Read the model definition and answer for the solid it produces. Units are mm, in the model's axes. Round coordinates to 2 decimals unless told otherwise and drop trailing zeros. Order: outer loops, then holes, each group sorted by start corner. A loop starts at its lowest first (then second) coordinate and runs counter-clockwise, first axis right, second up. Notation, with made-up numbers: (3.25, 62) - (57.25, 62) arc R23 ccw to (57.25, 85) - close; hole circle Ø6 at (61.25, -18). An arc over 180 degrees is marked (long way). Answer as a JSON object with one key per item and string values. Group by question number.
Q1. A cutting plane is placed at B-B on x = -267. Determine the outline of the cut face in (y, z).
Q2. Given pin 1 Ø22.5 at (y, z) = (-24.5, 271) entering from -X; pin 2 Ø1.5 at (x, y) = (-140.5, -14.5) entering from +Z; pin 3 Ø8 at (y, z) = (-28.5, 216) entering from +X, each flat-ended and moving along its own axis, determine where each tip first touches the part or whether it passes through.
Q3. A cutting plane is placed at D-D on z = 712.5. Determine the outline of the cut face in (x, y), and give its area (4 significant figures).
Q4. A cutting plane is placed at C-C on z = 258. Determine the outline of the cut face in (x, y), and give its area (3 significant figures).
Q5. A cutting plane is placed at A-A on y = -9.5. Determine the outline of the cut face in (x, z).
Q6. Consider line 1 (X direction, y = -27.5, z = 483.5); line 2 (Z direction, x = -178.5, y = -27); line 3 (Z direction, x = 104, y = -19). Determine where each line is inside the solid, lowest interval first.
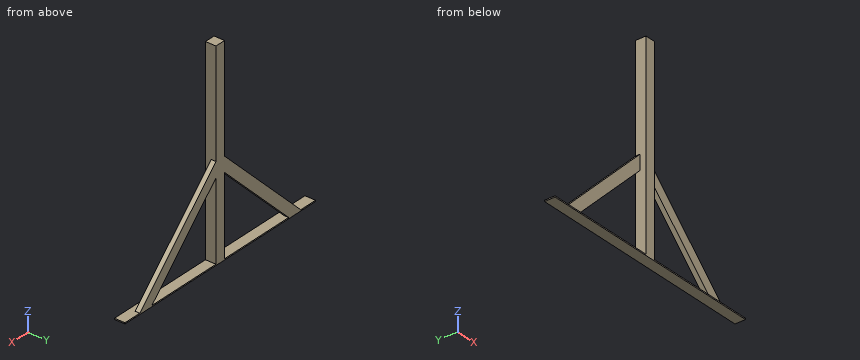
```python
from build123d import *

# Parameters (mm, degrees)
F1_DEPTH = 45
F2_DEPTH = 20


with BuildPart() as f1:
    # F0 (on Front) → F1 (new body)
    with BuildSketch(Plane.XZ):
        Polygon((22.5, 338.86039), (22.5, 402.5), (22.5, 852.5), (-22.5, 852.5), (-22.5, 402.133873), (-22.5, 338.86039), (-22.5, 2.5), (22.5, 2.5), align=None)
        Polygon((500, -2.5), (500, 2.5), (422.5, 2.5), (358.86039, 2.5), (22.5, 2.5), (-22.5, 2.5), (-359.168549, 2.5), (-422.5, 2.5), (-500, 2.5), (-500, -2.5), align=None)
    extrude(amount=F1_DEPTH)

    # F0 (on Front) → F2 (join)
    with BuildSketch(Plane.XZ):
        Polygon((500, -2.5), (500, 2.5), (422.5, 2.5), (358.86039, 2.5), (22.5, 2.5), (-22.5, 2.5), (-359.168549, 2.5), (-422.5, 2.5), (-500, 2.5), (-500, -2.5), align=None)
        Polygon((358.86039, 2.5), (422.5, 2.5), (22.5, 402.5), (22.5, 338.86039), align=None)
        Polygon((22.5, 338.86039), (22.5, 402.5), (22.5, 852.5), (-22.5, 852.5), (-22.5, 402.133873), (-22.5, 338.86039), (-22.5, 2.5), (22.5, 2.5), align=None)
        Polygon((-22.5, 402.133873), (-422.5, 2.5), (-359.168549, 2.5), (-22.5, 338.86039), align=None)
    extrude(amount=F2_DEPTH)


solid = f1.part
```
Result set:
{
 "1": {"outline": "(-45, -2.5) - (0, -2.5) - (0, 2.5) - (-45, 2.5) - close; (-20, 94.58) - (0, 94.58) - (0, 157.86) - (-20, 157.86) - close"},
 "2": {"pin 1": "stops at x = -164.07", "pin 2": "stops at z = 284.99", "pin 3": "stops at x = 22.5"},
 "3": {"outline": "(-22.5, -45) - (22.5, -45) - (22.5, 0) - (-22.5, 0) - close", "area": "2,025 mm²"},
 "4": {"outline": "(-166.77, -20) - (-103.43, -20) - (-103.43, 0) - (-166.77, 0) - close; (-22.5, -45) - (22.5, -45) - (22.5, 0) - (-22.5, 0) - close; (103.36, -20) - (167, -20) - (167, 0) - (103.36, 0) - close", "area": "4,560 mm²"},
 "5": {"outline": "(-500, -2.5) - (500, -2.5) - (500, 2.5) - (422.5, 2.5) - (22.5, 402.5) - (22.5, 852.5) - (-22.5, 852.5) - (-22.5, 402.13) - (-422.5, 2.5) - (-500, 2.5) - close; hole (-359.17, 2.5) - (-22.5, 2.5) - (-22.5, 338.86) - close; hole (22.5, 2.5) - (358.86, 2.5) - (22.5, 338.86) - close"},
 "6": {"line 1": "x = -22.5 to 22.5", "line 2": "z = -2.5 to 2.5", "line 3": "z = -2.5 to 2.5, 257.36 to 321"}
}
